The drawing under review shows one solid part. Ordinate dimensions are in mm from its lowest x, y, z. A direction names the side the tool comes from. Coordinates: 2 decimals unless noted, no trailing zeros. Write each loop counter-clockwise with the first axis right and the second up, starting at its lowest first coordinate (ties: lowest second). Pieces come first, ordered by that corner, then holes.
Q1. Insertion check: pin 1 (5 mm diameter, centred on y = 79.5, z = 99.5, fed in from +X); pin 2 (8 mm diameter, centred on y = 56, z = 18.5, fed in from -X); pin 3 (2 mm diameter, centred on y = 56.5, z = 101, fed in from +X); pin 4 (8 mm diameter, centred on x = 26.5, z = 83.5, fed in from +Y). Each pin has a flat end and moves straight along its axis. Give the tip position at first contact, or say it passes through.
Q2. Take a section at D-D (z = 69.5). Give the boundary of the cut face in (x, y).
Q3. Take a section at A-A (y = 51). Give the boundary of the cut face in (x, z).
Q4. For probe 1 along Z at (x, y) = (75.5, 64.5); probe 2 along Y at (x, z) = (8, 58); probe 3 along X at (y, z) = (36, 91), list the stretches that pass through material, from the lowest coordinate up.
Q5. Take a section at C-C (z = 101). Give the boundary of the cut face in (x, y), and give its area (3 significant figures).
Q6. Machinability: for the marked faces 1, 2 and 3, which of the approach directions +Z, -Z, +X, -X, +Y, -Y give a long, thin tool a straight path to every point of the face, cutting with its end or side? Answer none if there is none.
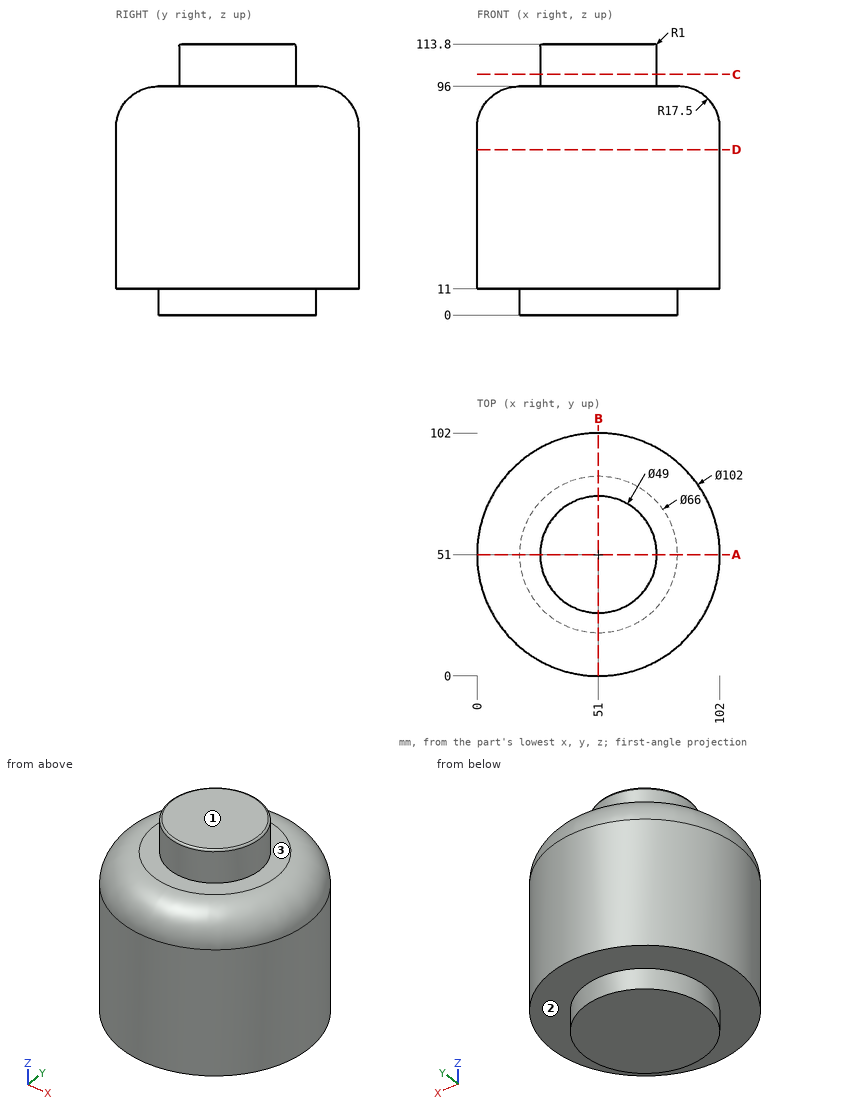
Response:
1. pin 1: passes through
1. pin 2: stops at x = 0.01
1. pin 3: stops at x = 75.08
1. pin 4: stops at y = 97.19
2. outline: circle Ø102 at (51, 51)
3. outline: (0, 11) - (18, 11) - (18, 0) - (84, 0) - (84, 11) - (102, 11) - (102, 78.5) arc R17.5 ccw to (84.5, 96) - (75.5, 96) - (75.5, 112.8) arc R1 ccw to (74.5, 113.8) - (27.5, 113.8) arc R1 ccw to (26.5, 112.8) - (26.5, 96) - (17.5, 96) arc R17.5 ccw to (0, 78.5) - close
4. probe 1: z = 0 to 96
4. probe 2: y = 23.58 to 78.42
4. probe 3: x = 7.78 to 94.22
5. outline: circle Ø49 at (51, 51)
5. area: 1,890 mm2
6. face 1: +Z, +X, -X, +Y, -Y
6. face 2: -Z
6. face 3: +Z
